```python
from build123d import *

# Parameters (mm, degrees)
SKETCH1_W               = 122
SKETCH1_H               = 110
BOSS_EXTRUDE1_DEPTH     = 11
SKETCH4_W               = 116
SKETCH4_H               = 104
CUT_EXTRUDE1_DEPTH      = 8
SKETCH6_R               = 1.999999993
SKETCH6_R_2             = 2
CUT_EXTRUDE6_DEPTH      = 120
CUT_EXTRUDE6_DEPTH_BACK = 4
SKETCH5_R               = 2
CUT_EXTRUDE5_DEPTH      = 108
CUT_EXTRUDE5_DEPTH_BACK = 4
FILLET2_R               = 1


with BuildPart() as part:
    # Sketch1 → Boss-Extrude1 (new body)
    with BuildSketch(Plane(origin=(0, 0, 0), x_dir=(1, 0, 0), z_dir=(0, 1, 0))):
        with Locations((-140.609907121, 22.894736842)):
            Rectangle(SKETCH1_W, SKETCH1_H)
    extrude(amount=BOSS_EXTRUDE1_DEPTH)

    # Sketch4 → Cut-Extrude1 (cut)
    with BuildSketch(Plane(origin=(0, 11, 0), x_dir=(1, 0, 0), z_dir=(0, 1, 0))):
        with Locations((-140.609907121, 22.894736842)):
            Rectangle(SKETCH4_W, SKETCH4_H)
    extrude(amount=-CUT_EXTRUDE1_DEPTH, mode=Mode.SUBTRACT)

    # Sketch6 → Cut-Extrude6 (cut, two sides)
    with BuildSketch(Plane(origin=(-198.609907121, 0, 0), x_dir=(0, 0, -1), z_dir=(1, 0, 0))) as cut_extrude6_sk:
        with Locations((-2.105263158, 6.999999977)):
            Circle(SKETCH6_R)
        with Locations((22.894736842, 6.999999977)):
            Circle(SKETCH6_R)
        with Locations((47.894736842, 7)):
            Circle(SKETCH6_R_2)
    extrude(amount=CUT_EXTRUDE6_DEPTH, mode=Mode.SUBTRACT)
    extrude(cut_extrude6_sk.sketch, amount=-CUT_EXTRUDE6_DEPTH_BACK, mode=Mode.SUBTRACT)

    # Sketch5 → Cut-Extrude5 (cut, two sides)
    with BuildSketch(Plane.XY.offset(-74.894736842)) as cut_extrude5_sk:
        with Locations((-169.359907121, 7)):
            Circle(SKETCH5_R)
        with Locations((-140.109907121, 7)):
            Circle(SKETCH5_R)
        with Locations((-110.859907121, 7)):
            Circle(SKETCH5_R)
    extrude(amount=CUT_EXTRUDE5_DEPTH, mode=Mode.SUBTRACT)
    extrude(cut_extrude5_sk.sketch, amount=-CUT_EXTRUDE5_DEPTH_BACK, mode=Mode.SUBTRACT)

    # Fillet2
    fillet2_edges = [part.edges().sort_by_distance(p)[0] for p in [
        (-79.609907121, 11, -22.894736842),
        (-140.609907121, 11, -77.894736842),
        (-198.609907121, 11, -22.894736842),
        (-140.609907121, 11, 29.105263158),
        (-82.609907121, 11, -22.894736842),
        (-140.609907121, 11, -74.894736842),
        (-201.609907121, 11, -22.894736842),
        (-140.609907121, 11, 32.105263158),
    ]]
    fillet(fillet2_edges, radius=FILLET2_R)


solid = part.part
```
Can you work these out from the model? Positions are in its coordinate system, mm. A direction names the side the tool comes from. Coordinates: 2 decimals unless noted, no trailing zeros. Loops run counter-clockwise (first coordinate to the right, second up) from the corner with the lowest first, then second, coordinate; pieces in that order, holes last.
Item 1: Suppose I cut it at D-D (z = -66.5). Please give me the cut outline in (x, y).
Answers below:
outline: (-201.61, 0) - (-79.61, 0) - (-79.61, 10) arc R1 ccw to (-80.61, 11) - (-81.61, 11) arc R1 ccw to (-82.61, 10) - (-82.61, 3) - (-198.61, 3) - (-198.61, 10) arc R1 ccw to (-199.61, 11) - (-200.61, 11) arc R1 ccw to (-201.61, 10) - close
Item 2: Suppose I cut it at B-B (x = -134). Please give me the cut outline in (y, z), then the cut area to 3 significant figures.
Answers below:
outline: (0, -77.89) - (10, -77.89) arc R1 ccw to (11, -76.89) - (11, -75.89) arc R1 ccw to (10, -74.89) - (3, -74.89) - (3, 29.11) - (10, 29.11) arc R1 ccw to (11, 30.11) - (11, 31.11) arc R1 ccw to (10, 32.11) - (0, 32.11) - close
area: 377 mm2
Item 3: Suppose I cut it at C-C (y = 7). State how many separate pieces and enclosed holes the cut face has, then the cut area to 3 significant figures.
Answers below:
separate pieces: 12
enclosed holes: 0
area: 1,210 mm2
Item 4: If we mould it in two halves opening along Y, with no side actions, what happens to faces 1 (the face through (-141, 5, 32.105)), 2 (the face through (-141, 0, -24)), 3 (the face through (-81.131, 5.048, 2.539))? For each: released by +Y, released by -Y, zero draft, split by the parting line, or undercut.
Answers below:
face 1: zero draft
face 2: released by -Y
face 3: undercut
Item 5: Which directions (+Z, -Z, +X, -X, +Y, -Y) give clear straight access to the entire face, cutting with the end or side of a thin tool? Please do faces 4 (the face through (-141, 5, 29.105)), 5 (the face through (-201.61, 5, -22)).
Answers below:
face 4: +Y
face 5: +Z, -Z, -X, +Y, -Y
Item 6: Suppose I cut it at A-A (z = -23). Please give me the cut outline in (x, y), then the cut area to 3 significant figures.
Answers below:
outline: (-201.61, 0) - (-79.61, 0) - (-79.61, 5) - (-82.61, 5) - (-82.61, 3) - (-198.61, 3) - (-198.61, 5) - (-201.61, 5) - close; (-201.61, 9) - (-198.61, 9) - (-198.61, 10) arc R1 ccw to (-199.61, 11) - (-200.61, 11) arc R1 ccw to (-201.61, 10) - close; (-82.61, 9) - (-79.61, 9) - (-79.61, 10) arc R1 ccw to (-80.61, 11) - (-81.61, 11) arc R1 ccw to (-82.61, 10) - close
area: 389 mm2
Item 7: Please list where these lines run through material, in increasing order: L1, parallel to X at y = 7, z = 30; L2, parallel to Z at x = -84.5, y = 3.5; L3, parallel to X at y = 7.5, z = -6.
Answers below:
L1: x = -201.61 to -171.36, -167.36 to -142.11, -138.11 to -112.86, -108.86 to -79.61
L2: z = -77.89 to -74.89, 29.11 to 32.11
L3: x = -201.61 to -198.61, -82.61 to -79.61
